Print and shaded views of the part. All mm, measured from the part's lowest x, y and z. A direction names the side the tool comes from. Give positions to 0.01 mm unless a question says otherwise; leave off trailing zeros. Write each loop counter-clockwise with the first axis right and the second up, starting at its lowest first coordinate (ties: lowest second). Pieces come first, ordered by that corner, then holes.
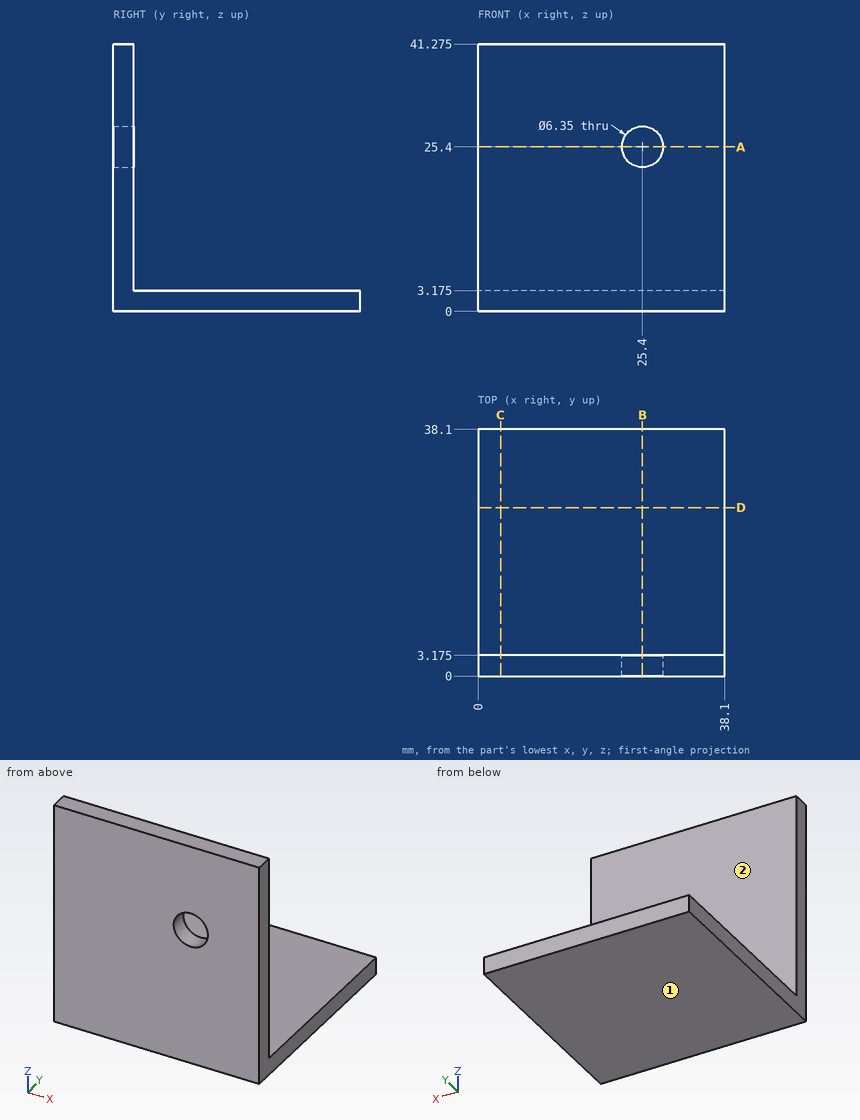
1. Saw through at D-D on y = 26. Give the cut face in (x, z) (3 decimals), plus the area to 3 significant figures.
2. Saw through at C-C on x = 3.5. Give the cut face in (y, z) (3 decimals).
3. Saw through at B-B on x = 25.4. Give the cut face in (y, z) (3 decimals).
4. Drop flat-ended pins along their axis: pin 1 (1.5 mm diameter, centred on x = 32, y = 8.5, fed in from +Z) (3 decimals); pin 2 (11.5 mm diameter, centred on x = 25.5, z = 31, fed in from +Y) (3 decimals). Give the stop position or say it passes through.
5. 3-axis set-ups, long thin cutter, end or side, ignore diameter. For the marked faces 1 and 2: which of +Z, -Z, +X, -X, +Y, -Y reach the whole face in a straight line?
6. Saw through at A-A on z = 25.4. Give the cut face in (x, y) (3 decimals).
7. Drill centre lines: line 1 along X through (y, z) = (1.35, 25.4) (3 decimals); line 2 along Z through (x, y) = (25.4, 1.9) (3 decimals); line 3 along Y through (x, z) = (9, 15.5) (3 decimals). Where is each one in solid material? Low to high.
Outcome:
1. outline: (0, 0) - (38.1, 0) - (38.1, 3.175) - (0, 3.175) - close
1. area: 121 mm2
2. outline: (0, 0) - (38.1, 0) - (38.1, 3.175) - (3.175, 3.175) - (3.175, 41.275) - (0, 41.275) - close
3. outline: (0, 0) - (38.1, 0) - (38.1, 3.175) - (3.175, 3.175) - (3.175, 22.225) - (0, 22.225) - close; (0, 28.575) - (3.175, 28.575) - (3.175, 41.275) - (0, 41.275) - close
4. pin 1: stops at z = 3.175
4. pin 2: stops at y = 3.175
5. face 1: -Z, +X, -X, +Y, -Y
5. face 2: +Z, +X, -X, +Y
6. outline: (0, 0) - (22.225, 0) - (22.225, 3.175) - (0, 3.175) - close; (28.575, 0) - (38.1, 0) - (38.1, 3.175) - (28.575, 3.175) - close
7. line 1: x = 0 to 22.225, 28.575 to 38.1
7. line 2: z = 0 to 22.225, 28.575 to 41.275
7. line 3: y = 0 to 3.175
